```python
from build123d import *

# Parameters (mm, degrees)
SKETCH1_R           = 8
SKETCH1_R_2         = 1.5
SKETCH1_R_3         = 1.25
BOSS_EXTRUDE1_DEPTH = 1.5


with BuildPart() as part:
    # Sketch1 → Boss-Extrude1 (new body)
    with BuildSketch(Plane.XY):
        with BuildLine():
            Line((-22.075, -25.075), (22.075, -25.075))
            ThreePointArc((22.075, -25.075), (24.196320344, -24.196320344), (25.075, -22.075))
            Line((25.075, -22.075), (25.075, 22.075))
            ThreePointArc((25.075, 22.075), (24.196320344, 24.196320344), (22.075, 25.075))
            Line((22.075, 25.075), (-22.075, 25.075))
            ThreePointArc((-22.075, 25.075), (-24.196320344, 24.196320344), (-25.075, 22.075))
            Line((-25.075, 22.075), (-25.075, -22.075))
            ThreePointArc((-25.075, -22.075), (-24.196320344, -24.196320344), (-22.075, -25.075))
        make_face()
        Circle(SKETCH1_R, mode=Mode.SUBTRACT)
        with Locations((-22.605330086, 22.605330086)):
            Circle(SKETCH1_R_2, mode=Mode.SUBTRACT)
        with Locations(Location((22.605330086, -22.605330086, 0), (0, 0, 180))):
            Circle(SKETCH1_R_2, mode=Mode.SUBTRACT)
        with Locations((22.605330086, 22.605330086)):
            Circle(SKETCH1_R_2, mode=Mode.SUBTRACT)
        with Locations(Location((-22.605330086, -22.605330086, 0), (0, 0, 180))):
            Circle(SKETCH1_R_2, mode=Mode.SUBTRACT)
        with Locations((-17.655582618, 17.655582618)):
            Circle(SKETCH1_R_2, mode=Mode.SUBTRACT)
        with Locations(Location((17.655582618, -17.655582618, 0), (0, 0, 180))):
            Circle(SKETCH1_R_2, mode=Mode.SUBTRACT)
        with Locations((17.655582618, 17.655582618)):
            Circle(SKETCH1_R_2, mode=Mode.SUBTRACT)
        with Locations(Location((-17.655582618, -17.655582618, 0), (0, 0, 180))):
            Circle(SKETCH1_R_2, mode=Mode.SUBTRACT)
        with Locations((-3.75, 22.05)):
            Circle(SKETCH1_R_3, mode=Mode.SUBTRACT)
        with Locations((3.75, 22.05)):
            Circle(SKETCH1_R_3, mode=Mode.SUBTRACT)
        with Locations((11.25, 22.05)):
            Circle(SKETCH1_R_3, mode=Mode.SUBTRACT)
        with Locations((-11.25, 22.05)):
            Circle(SKETCH1_R_3, mode=Mode.SUBTRACT)
        with Locations(Location((11.25, -22.05, 0), (0, 0, 180))):
            Circle(SKETCH1_R_3, mode=Mode.SUBTRACT)
        with Locations(Location((3.75, -22.05, 0), (0, 0, 180))):
            Circle(SKETCH1_R_3, mode=Mode.SUBTRACT)
        with Locations(Location((-3.75, -22.05, 0), (0, 0, 180))):
            Circle(SKETCH1_R_3, mode=Mode.SUBTRACT)
        with Locations(Location((-11.25, -22.05, 0), (0, 0, 180))):
            Circle(SKETCH1_R_3, mode=Mode.SUBTRACT)
        with Locations(Location((-22.05, 3.75, 0), (0, 0, 180))):
            Circle(SKETCH1_R_3, mode=Mode.SUBTRACT)
        with Locations(Location((-22.05, 11.25, 0), (0, 0, 180))):
            Circle(SKETCH1_R_3, mode=Mode.SUBTRACT)
        with Locations((-22.05, -11.25)):
            Circle(SKETCH1_R_3, mode=Mode.SUBTRACT)
        with Locations((-22.05, -3.75)):
            Circle(SKETCH1_R_3, mode=Mode.SUBTRACT)
        with Locations(Location((22.05, -11.25, 0), (0, 0, 180))):
            Circle(SKETCH1_R_3, mode=Mode.SUBTRACT)
        with Locations(Location((22.05, -3.75, 0), (0, 0, 180))):
            Circle(SKETCH1_R_3, mode=Mode.SUBTRACT)
        with Locations((22.05, 3.75)):
            Circle(SKETCH1_R_3, mode=Mode.SUBTRACT)
        with Locations((22.05, 11.25)):
            Circle(SKETCH1_R_3, mode=Mode.SUBTRACT)
        with Locations((-11.25, 15.55)):
            Circle(SKETCH1_R_2, mode=Mode.SUBTRACT)
        with Locations((-3.75, 15.55)):
            Circle(SKETCH1_R_2, mode=Mode.SUBTRACT)
    extrude(amount=BOSS_EXTRUDE1_DEPTH)


solid = part.part
```
The listing builds one solid part. Answer for the finished solid, in the listing's coordinates (mm). Give positions to 0.01 mm unless a question says otherwise; leave off trailing zeros. Loops run counter-clockwise (first coordinate to the right, second up) from the corner with the lowest first, then second, coordinate; pieces in that order, holes last. Notation, with made-up numbers: (-20.75, 83) - (-9.75, 83) arc R19 cw to (-9.75, 114) - close; hole circle Ø9 at (45.25, 54.5). An arc over 180 degrees is marked (long way). Answer as CSV lines item,"result". Start each with the question number.
Item 1: Find the intervals of material crossed by line 1 (X direction, y = -17.5, z = 0.6) (1 decimal); line 2 (Y direction, x = -16.5, z = 0.85) (3 decimals); line 3 (X direction, y = 3, z = 0.3) (3 decimals), in increasing order. Write a range as from..to.
Item 2: A cutting plane is placed at A-A on x = 11.25. Determine the outline of the cut face in (y, z) (3 decimals).
Item 3: The mould has two halves that part along X. Classify faces 1 (the face through (24.22, 24.17, 0.74)), 2 (the face through (0, -25.075, 1)), 3 (the face through (3.48, 20.83, 0.74)): +X half, -X half, draft (parallel to the pull), parting line (faces both ways), or undercut.
Item 4: Each of these flat-tipped pins is pushed along its axis until it touches: pin 1 (1.5 mm diameter, centred on x = 22.05, y = 11.25, fed in from -Z); pin 2 (8 mm diameter, centred on x = -19.5, y = -13.5, fed in from -Z). Where does it stop, or does it pass through?
Item 5: A cutting plane is placed at C-C on x = -4. Determine the outline of the cut face in (y, z) (3 decimals), then the cut area to 3 significant figures.
Item 6: A cutting plane is placed at D-D on y = -1. Determine the outline of the cut face in (x, z) (3 decimals).
Found:
1,line 1,"x = -25.1..-19.1, -16.2..16.2, 19.1..25.1"
1,line 2,"y = -25.075..-18.612, -16.699..16.699, 18.612..25.075"
1,line 3,"x = -25.075..-23.05, -21.05..-7.416, 7.416..21.05, 23.05..25.075"
2,outline,"(-25.075, 0) - (-23.3, 0) - (-23.3, 1.5) - (-25.075, 1.5) - close; (-20.8, 0) - (20.8, 0) - (20.8, 1.5) - (-20.8, 1.5) - close; (23.3, 0) - (25.075, 0) - (25.075, 1.5) - (23.3, 1.5) - close"
3,face 1,"+X half"
3,face 2,"draft"
3,face 3,"undercut"
4,pin 1,"passes through"
4,pin 2,"stops at z = 0"
5,outline,"(-25.075, 0) - (-23.275, 0) - (-23.275, 1.5) - (-25.075, 1.5) - close; (-20.825, 0) - (-6.928, 0) - (-6.928, 1.5) - (-20.825, 1.5) - close; (6.928, 0) - (14.071, 0) - (14.071, 1.5) - (6.928, 1.5) - close; (17.029, 0) - (20.825, 0) - (20.825, 1.5) - (17.029, 1.5) - close; (23.275, 0) - (25.075, 0) - (25.075, 1.5) - (23.275, 1.5) - close"
5,area,"42.7 mm^2"
6,outline,"(-25.075, 0) - (-7.937, 0) - (-7.937, 1.5) - (-25.075, 1.5) - close; (7.937, 0) - (25.075, 0) - (25.075, 1.5) - (7.937, 1.5) - close"
